The model under review builds one solid part; all positions refer to its coordinate system, in mm. A direction names the side the tool comes from. Coordinates: 2 decimals unless noted, no trailing zeros. Order: outer loops, then holes, each group sorted by start corner. A loop starts at its lowest first (then second) coordinate and runs counter-clockwise, first axis right, second up. Notation, with made-up numbers: (-39.75, -32) -> (-21.75, -32) arc R25 ccw to (-21.75, -10) -> close; hole circle Ø7 at (22, 69.5). An arc over 180 degrees is marked (long way). Put each result on its own line as item: value.
from build123d import *

# Parameters (mm, degrees)
BOSS_EXTRUDE2_DEPTH = 40
SKETCH4_W           = 20
SKETCH4_H           = 15
CUT_EXTRUDE1_DEPTH  = 10
SKETCH5_R           = 7.5
CUT_EXTRUDE2_DEPTH  = 13


with BuildPart() as part:
    # Sketch2 → Boss-Extrude2 (new body)
    with BuildSketch(Plane.XY):
        with BuildLine():
            Line((0, 10), (0, 50))
            Line((0, 50), (10, 50))
            Line((10, 50), (10, 20))
            ThreePointArc((10, 20), (12.928932188, 12.928932188), (20, 10))
            Line((20, 10), (50, 10))
            Line((50, 10), (50, 0))
            Line((50, 0), (10, 0))
            ThreePointArc((10, 0), (2.928932188, 2.928932188), (0, 10))
        make_face()
    extrude(amount=BOSS_EXTRUDE2_DEPTH)

    # Sketch4 → Cut-Extrude1 (cut)
    with BuildSketch(Plane(origin=(0, 0, 0), x_dir=(0, 0, -1), z_dir=(1, 0, 0))):
        with Locations((-30, 42.5)):
            Rectangle(SKETCH4_W, SKETCH4_H)
    extrude(amount=CUT_EXTRUDE1_DEPTH, mode=Mode.SUBTRACT)

    # Sketch5 → Cut-Extrude2 (cut)
    with BuildSketch(Plane(origin=(0, 0, 0), x_dir=(1, 0, 0), z_dir=(0, 1, 0))):
        with Locations((35, -20)):
            Circle(SKETCH5_R)
        Polygon((35, -20), (35, -12.5), (50, -12.5), (50, -27.5), (35, -27.5), align=None)
    extrude(amount=CUT_EXTRUDE2_DEPTH, mode=Mode.SUBTRACT)


solid = part.part
Item 1: For pin 1 Ø6 at (x, z) = (27.5, 7.5) entering from +Y; pin 2 Ø5 at (x, z) = (5.5, 30) entering from +Y; pin 3 Ø11 at (x, y) = (7.5, 44.5) entering from +Z; pin 4 Ø8 at (x, y) = (34, 16.5) entering from -Z, all flat-tipped, find the tip position at first contact; note any pin that passes through.
Answers below:
pin 1: y = 10
pin 2: y = 35
pin 3: z = 20
pin 4: through
Item 2: Consider section B-B on z = 10.5. Write out the cut boundary in (x, y).
Answers below:
outline: (0, 10) arc R10 ccw to (10, 0) -> (50, 0) -> (50, 10) -> (20, 10) arc R10 cw to (10, 20) -> (10, 50) -> (0, 50) -> close
Item 3: For line 1 (Z direction, x = 44.5, y = 7); line 2 (Y direction, x = 27.5, z = 4), list the stretches that pass through material, from the lowest coordinate up. Write a range as from..to.
Answers below:
line 1: 0..12.5, 27.5..40
line 2: 0..10
Item 4: Consider section A-A on x = 40. Write out the cut boundary in (y, z), and give its area (3 significant figures).
Answers below:
outline: (0, 0) -> (10, 0) -> (10, 12.5) -> (0, 12.5) -> close; (0, 27.5) -> (10, 27.5) -> (10, 40) -> (0, 40) -> close
area: 250 mm^2
Item 5: Mouldability with a two-part tool opening along Z and no side actions: class faces 1 (the flat face through (5, 42, 20)), 2 (the flat face through (43, 5, 27.5)), 3 (the flat face through (42, 5, 12.5)), 4 (the flat face through (0, 25, 20)) as +Z half, -Z half, draft (parallel to the pull), parting line (faces both ways), or undercut.
Answers below:
face 1: +Z half
face 2: undercut
face 3: undercut
face 4: draft
Item 6: Consider section C-C on y = 39. Write out the cut boundary in (x, z), and give its area (3 significant figures).
Answers below:
outline: (0, 0) -> (10, 0) -> (10, 20) -> (0, 20) -> close
area: 200 mm^2
Item 7: Consider section D-D on x = 4. Write out the cut boundary in (y, z).
Answers below:
outline: (2, 0) -> (50, 0) -> (50, 20) -> (35, 20) -> (35, 40) -> (2, 40) -> close
Item 8: For faces 5 (the cylindrical face through (3.01, 2.85, 19.72)), 6 (the flat face through (10, 32, 15)), 7 (the flat face through (5, 35, 30)), list the 3-axis set-ups (+Z, -Z, +X, -X, +Y, -Y) from which the entire face can be reached by the end or side of a thin tool; tool diameter is ignored.
Answers below:
face 5: +Z, -Z, -X, -Y
face 6: +Z, -Z, +X, +Y
face 7: +Z, +X, -X, +Y
